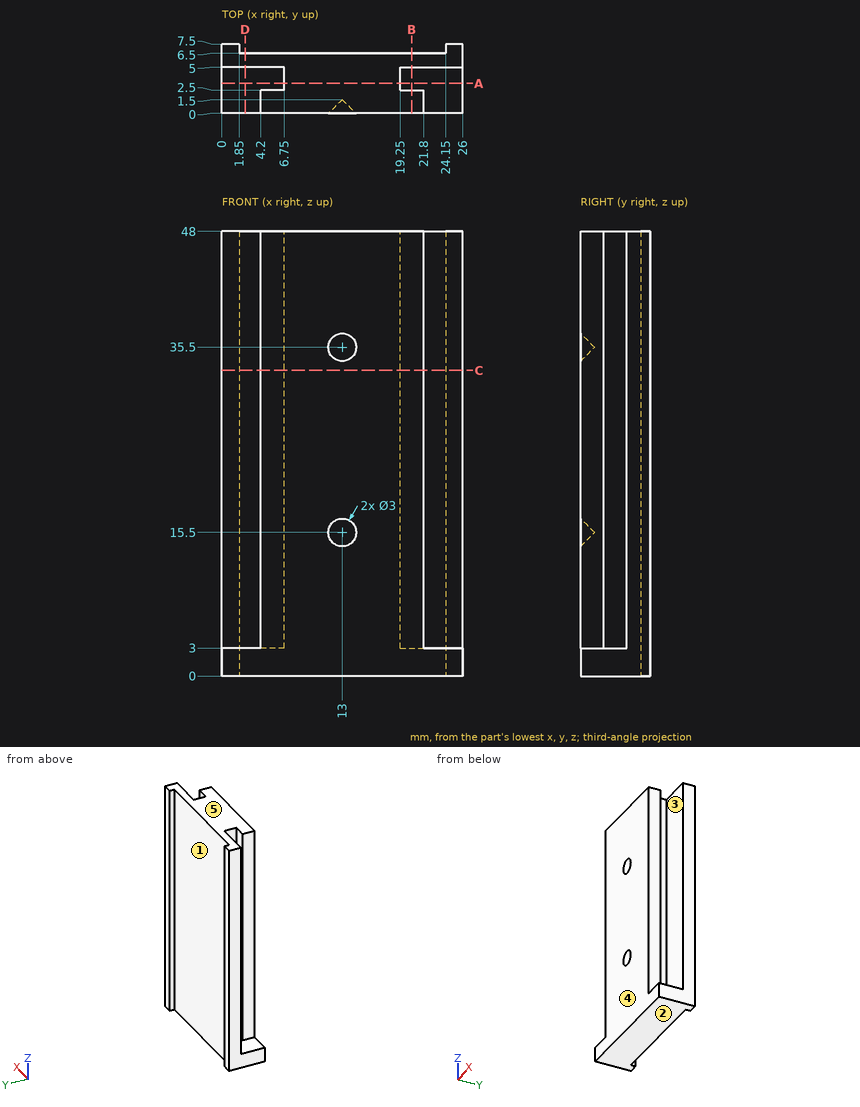
Print and shaded views of the part. All mm, measured from the part's lowest x, y and z. A direction names the side the tool comes from. Give positions to 0.01 mm unless a question says otherwise; leave off trailing zeros. Loops run counter-clockwise (first coordinate to the right, second up) from the corner with the lowest first, then second, coordinate; pieces in that order, holes last.
1) Flat gauge pins, fed straight in: pin 1 Ø1.2 at (y, z) = (1, 21) entering from -X; pin 2 Ø4 at (x, y) = (23, 3) entering from -Z; pin 3 Ø1.2 at (y, z) = (1, 20.5) entering from +X; pin 4 Ø1.3 at (x, z) = (20, 21.5) entering from +Y. Where does each tip first touch, or does it go through?
2) Saw through at A-A (y = 3.25). Write the cut outline in (x, z), plus the area to 4 significant figures.
3) Wall check: line 1 (Y direction, x = 19.75, z = 27.5); line 2 (X direction, y = 6.75, z = 42); line 3 (X direction, y = 4.75, z = 22.5). Give the ranges that are in metal, low to high.
4) Saw through at B-B (x = 20.5). Write the cut outline in (y, z), plus the area to 4 significant figures.
5) Tool access for the marked faces 1 and 2: list every direction of +Z, -Z, +X, -X, +Y, -Y with a clear straight run to the whole face (end or side of a thin tool).
6) Pull direction Y, two halves, no side cores. Call the marked faces 3, 4 and 5: +Y half, -Y half, draft (parallel to the pull), parting line (faces both ways), or undercut.
7) Saw through at C-C (z = 33). Write the cut outline in (x, y), plus the area to 3 significant figures.
8) Saw through at D-D (x = 2.5). Write the cut outline in (y, z).
Answer block:
1. pin 1: stops at x = 4.2
1. pin 2: stops at z = 0
1. pin 3: stops at x = 21.8
1. pin 4: stops at y = 6.5
2. outline: (0, 0) - (26, 0) - (26, 3) - (19.25, 3) - (19.25, 48) - (6.75, 48) - (6.75, 3) - (0, 3) - close
2. area: 640.5 mm2
3. line 1: y = 0 to 2.5, 5 to 6.5
3. line 2: x = 0 to 1.85, 24.15 to 26
3. line 3: x = 6.75 to 19.25
4. outline: (0, 0) - (6.5, 0) - (6.5, 48) - (5, 48) - (5, 3) - (2.5, 3) - (2.5, 48) - (0, 48) - close
4. area: 199.5 mm2
5. face 1: +Z, -Z, +Y
5. face 2: -Z, +X, -X, +Y, -Y
6. face 3: undercut
6. face 4: -Y half
6. face 5: draft
7. outline: (0, 5) - (6.75, 5) - (6.75, 2.5) - (4.2, 2.5) - (4.2, 0) - (21.8, 0) - (21.8, 2.5) - (19.25, 2.5) - (19.25, 5) - (26, 5) - (26, 7.5) - (24.15, 7.5) - (24.15, 6.5) - (1.85, 6.5) - (1.85, 7.5) - (0, 7.5) - close
7. area: 118 mm2
8. outline: (0, 0) - (6.5, 0) - (6.5, 48) - (5, 48) - (5, 3) - (0, 3) - close
